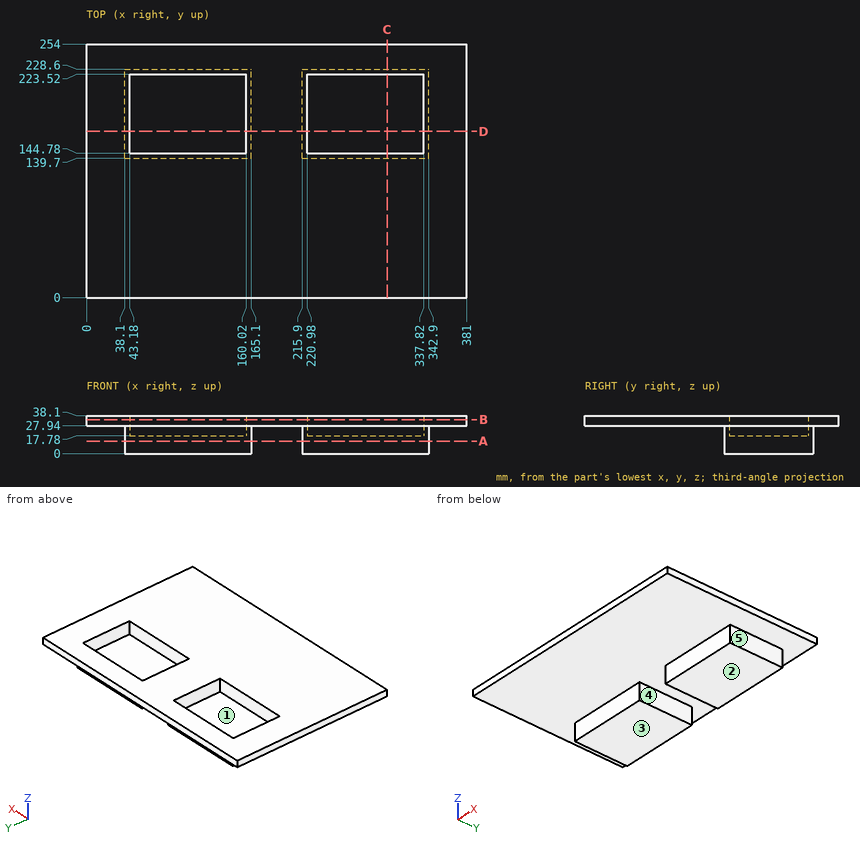
Job drawing, mm, ordinate dimensions from the low corner. One solid piece. A direction names the side the tool comes from. Give positions to 0.01 mm unless a question says otherwise; leave off trailing zeros. Loops run counter-clockwise (first coordinate to the right, second up) from the corner with the lowest first, then second, coordinate; pieces in that order, holes last. Notation, with made-up numbers: M 50,34.5 L 86,34.5 A15 cw 86,41.5 Z; hole C -14,51 d11. An arc over 180 degrees is marked long. Return JSON: item names as keys, results as strings.
1) Saw through at B-B, the plane z = 34. List the corners of the cut face in (x, y), then the cut area to 3 significant figures.
Calculated:
{"outline": "M 0,0 L 381,0 L 381,254 L 0,254 Z; hole M 43.18,144.78 L 160.02,144.78 L 160.02,223.52 L 43.18,223.52 Z; hole M 220.98,144.78 L 337.82,144.78 L 337.82,223.52 L 220.98,223.52 Z", "area": "78,400 mm2"}
2) 3-axis set-ups, long thin cutter, end or side, ignore diameter. For the marked faces 1 and 2: which of +Z, -Z, +X, -X, +Y, -Y reach the whole face in a straight line?
Calculated:
{"face 1": "+Z", "face 2": "-Z, +X, -X, +Y, -Y"}
3) Saw through at D-D, the plane y = 166.5. List the corners of the cut face in (x, z), then the cut area to 3 significant figures.
Calculated:
{"outline": "M 0,27.94 L 38.1,27.94 L 38.1,0 L 165.1,0 L 165.1,27.94 L 215.9,27.94 L 215.9,0 L 342.9,0 L 342.9,27.94 L 381,27.94 L 381,38.1 L 337.82,38.1 L 337.82,17.78 L 220.98,17.78 L 220.98,38.1 L 160.02,38.1 L 160.02,17.78 L 43.18,17.78 L 43.18,38.1 L 0,38.1 Z", "area": "6,220 mm2"}
4) Pull direction X, two halves, no side cores. Call the marked faces 3, 4 and 5: released by +X, released by -X, zero draft, split by the parting line, or undercut.
Calculated:
{"face 3": "zero draft", "face 4": "undercut", "face 5": "released by +X"}
5) Saw through at A-A, the plane z = 12.5. List the corners of the cut face in (x, y), then the cut area to 3 significant figures.
Calculated:
{"outline": "M 38.1,139.7 L 165.1,139.7 L 165.1,228.6 L 38.1,228.6 Z; M 215.9,139.7 L 342.9,139.7 L 342.9,228.6 L 215.9,228.6 Z", "area": "22,600 mm2"}
6) Saw through at C-C, the plane x = 301. List the corners of the cut face in (y, z), then the cut area to 3 significant figures.
Calculated:
{"outline": "M 0,27.94 L 139.7,27.94 L 139.7,0 L 228.6,0 L 228.6,27.94 L 254,27.94 L 254,38.1 L 223.52,38.1 L 223.52,17.78 L 144.78,17.78 L 144.78,38.1 L 0,38.1 Z", "area": "3,460 mm2"}
7) Drill centre lines: line 1 (Y direction, x = 124.5, z = 18); line 2 (X direction, y = 151, z = 16.5); line 3 (Y direction, x = 65, z = 30). Where is each one in solid material? Low to high.
Calculated:
{"line 1": "y = 139.7 to 144.78, 223.52 to 228.6", "line 2": "x = 38.1 to 165.1, 215.9 to 342.9", "line 3": "y = 0 to 144.78, 223.52 to 254"}
8) Flat gauge pins, fed straight in: pin 1 Ø3 at (y, z) = (190.5, 27.5) entering from -X; pin 2 Ø14 at (x, z) = (267.5, 8) entering from +Y; pin 3 Ø1.5 at (y, z) = (172.5, 20) entering from -X; pin 4 Ø6 at (x, z) = (90, 13) entering from -Y. Where does each tip first touch, or does it go through?
Calculated:
{"pin 1": "stops at x = 0", "pin 2": "stops at y = 228.6", "pin 3": "stops at x = 38.1", "pin 4": "stops at y = 139.7"}
